Work out the finished part from the listing and answer in its coordinate system (mm). A direction names the side the tool comes from. Round coordinates to 2 decimals unless told otherwise and drop trailing zeros. Order: outer loops, then holes, each group sorted by start corner. A loop starts at its lowest first (then second) coordinate and runs counter-clockwise, first axis right, second up. Notation, with made-up numbers: (-4.5, 54.25) -> (43.5, 54.25) arc R26 cw to (43.5, 77.25) -> close; hole circle Ø9 at (22, 23). An arc over 180 degrees is marked (long way). Use one line per item in the form item = value.
```python
from build123d import *

# Parameters (mm, degrees)
SKETCH_1_R          = 12
SKETCH_1_R_2        = 4
EXTRUDE_1_DEPTH     = 2
SKETCH_2_R          = 6
SKETCH_2_R_2        = 4
EXTRUDE_3_DEPTH     = 10
SKETCH_4_R          = 1.75
CUT_EXTRUDE_1_DEPTH = 16.7


with BuildPart() as part:
    # 草图1 → 凸台-拉伸1 (new body)
    with BuildSketch(Plane.XY):
        Circle(SKETCH_1_R)
        Circle(SKETCH_1_R_2, mode=Mode.SUBTRACT)
    extrude(amount=EXTRUDE_1_DEPTH)

    # 草图2 → 凸台-拉伸3 (add)
    with BuildSketch(Plane.XY.offset(2)):
        Circle(SKETCH_2_R)
        Circle(SKETCH_2_R_2, mode=Mode.SUBTRACT)
    extrude(amount=EXTRUDE_3_DEPTH)

    # 草图4 → 切除-拉伸1 (cut)
    with BuildSketch(Plane(origin=(0, 0, 0), x_dir=(-1, 0, 0), z_dir=(0, 0, -1))):
        with Locations((9, 0)):
            Circle(SKETCH_4_R)
        with Locations((0, 9)):
            Circle(SKETCH_4_R)
        with Locations((-9, 0)):
            Circle(SKETCH_4_R)
        with Locations((0, -9)):
            Circle(SKETCH_4_R)
    extrude(amount=-CUT_EXTRUDE_1_DEPTH, mode=Mode.SUBTRACT)


solid = part.part
```
Item 1: Consider line 1 along Y through (x, z) = (0, 1.15); line 2 along Y through (x, z) = (0, 5.5); line 3 along X through (y, z) = (-0.25, 1.5). Determine where each line is inside the solid, lowest interval first.
Findings:
line_1 = -12 to -10.75, -7.25 to -4, 4 to 7.25, 10.75 to 12
line_2 = -6 to -4, 4 to 6
line_3 = -12 to -10.73, -7.27 to -3.99, 3.99 to 7.27, 10.73 to 12
Item 2: Determine the mould class of faces 1 (the flat face through (-3, 3, 0)), 2 (the cylindrical face through (-11.99, 0.53, 0.99)), 3 (the cylindrical face through (0.228, -7.265, 0.986)) for opening direction X: released by +X, released by -X, zero draft, split by the parting line, or undercut.
Findings:
face_1 = zero draft
face_2 = split by the parting line
face_3 = undercut
Item 3: The part is cut by section B-B, the plane y = 9. Give the vertices of the cut face in (x, z), and give its area (3 significant figures).
Findings:
outline = (-7.94, 0) -> (-1.75, 0) -> (-1.75, 2) -> (-7.94, 2) -> close; (1.75, 0) -> (7.94, 0) -> (7.94, 2) -> (1.75, 2) -> close
area = 24.7 mm^2
Item 4: Flat-ended cylindrical pins translate along their axes: P1, Ø6, axis at x = 8.5, y = 8, coming from the +Z side; P2, Ø2, axis at y = 2.5, z = 6.5, coming from the -X side; P3, Ø1.5, axis at x = -5, z = 6, coming from the +Y side. Find the tip coordinate at first contact, or state that the pin passes through.
Findings:
P1 = 2
P2 = -5.81
P3 = 4.24
Item 5: For faces 4 (the flat face through (-1.42, -3.92, 12)), 5 (the cylindrical face through (-6, 0, 7)), determine the directions among +Z, -Z, +X, -X, +Y, -Y from which every point of the face is accessible in a straight line to the end or side of a thin tool.
Findings:
face_4 = +Z, +X, -X, +Y, -Y
face_5 = +Z
Item 6: The part is cut by section A-A, the plane x = 0. Give the vertices of the cut face in (y, z).
Findings:
outline = (-12, 0) -> (-10.75, 0) -> (-10.75, 2) -> (-12, 2) -> close; (-7.25, 0) -> (-4, 0) -> (-4, 12) -> (-6, 12) -> (-6, 2) -> (-7.25, 2) -> close; (4, 0) -> (7.25, 0) -> (7.25, 2) -> (6, 2) -> (6, 12) -> (4, 12) -> close; (10.75, 0) -> (12, 0) -> (12, 2) -> (10.75, 2) -> close
